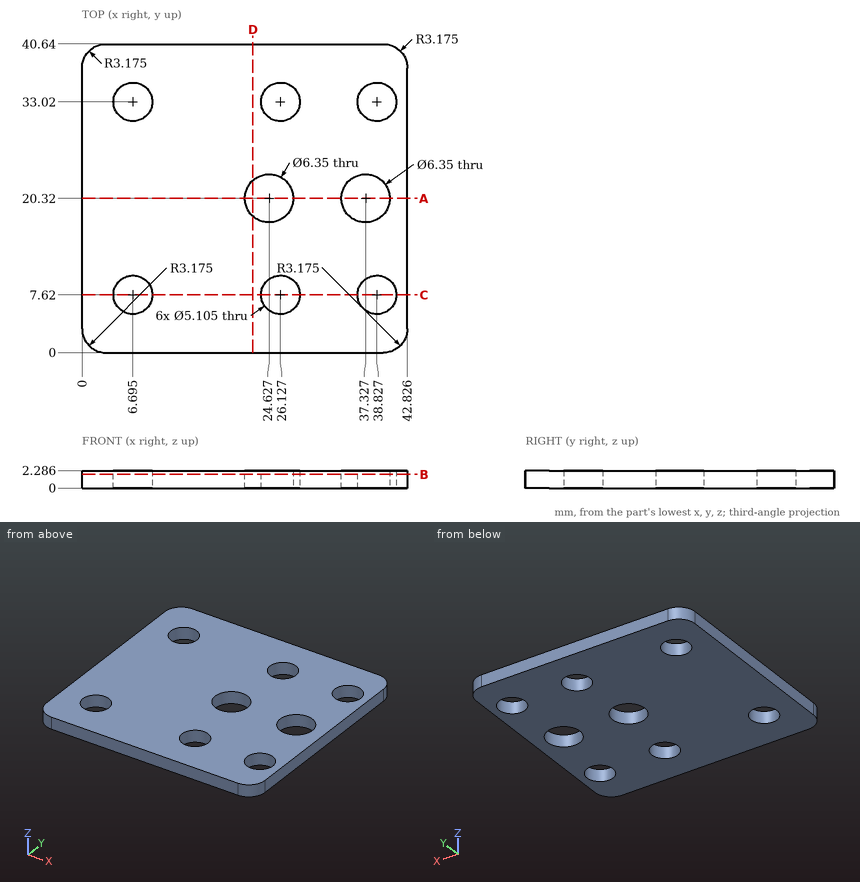
Part print with two shaded views. Sizes in mm from the minimum x, y, z corner. Coordinates: 2 decimals unless noted, no trailing zeros. Write each loop counter-clockwise with the first axis right and the second up, starting at its lowest first coordinate (ties: lowest second). Pieces come first, ordered by that corner, then holes. Notation, with made-up numbers: (-34.5, -34) -> (14.5, -34) arc R16 cw to (14.5, -25) -> close; hole circle Ø11 at (86.5, 44). An arc over 180 degrees is marked (long way). Return JSON: item names as keys, results as strings. Group by question number.
Q1. Cut at B-B, the plane z = 1.8. State how many separate pieces and enclosed holes the cut face has, then the cut area to 3 significant figures.
Q2. Cut at A-A, the plane y = 20.32. Give the cut face in (x, z) (1 decimal).
Q3. Flat gauge pin, fed straight in: pin 1 (3 mm diameter, centred on x = 26.13, y = 33.02, fed in from +Z). Where does the tip first touch, or does it go through?
Q4. Cut at C-C, the plane y = 7.62. Give the cut face in (x, z) (1 decimal).
Q5. Drill centre lines: line 1 (X direction, y = 20.32, z = 1.45) (1 decimal); line 2 (X direction, y = 34.5, z = 1.6) (1 decimal); line 3 (Y direction, x = 27.5, z = 1.9) (1 decimal). Where is each one in solid material? Low to high.
Q6. Cut at D-D, the plane x = 22.5. Give the cut face in (y, z).
Returned:
{
 "1": {"separate pieces": "1", "enclosed holes": "8", "area": "1,550 mm2"},
 "2": {"outline": "(0, 0) -> (21.5, 0) -> (21.5, 2.3) -> (0, 2.3) -> close; (27.8, 0) -> (34.2, 0) -> (34.2, 2.3) -> (27.8, 2.3) -> close; (40.5, 0) -> (42.8, 0) -> (42.8, 2.3) -> (40.5, 2.3) -> close"},
 "3": {"pin 1": "passes through"},
 "4": {"outline": "(0, 0) -> (4.1, 0) -> (4.1, 2.3) -> (0, 2.3) -> close; (9.2, 0) -> (23.6, 0) -> (23.6, 2.3) -> (9.2, 2.3) -> close; (28.7, 0) -> (36.3, 0) -> (36.3, 2.3) -> (28.7, 2.3) -> close; (41.4, 0) -> (42.8, 0) -> (42.8, 2.3) -> (41.4, 2.3) -> close"},
 "5": {"line 1": "x = 0 to 21.5, 27.8 to 34.2, 40.5 to 42.8", "line 2": "x = 0 to 4.6, 8.8 to 24, 28.2 to 36.7, 40.9 to 42.8", "line 3": "y = 0 to 5.5, 9.8 to 19, 21.7 to 30.9, 35.2 to 40.6"},
 "6": {"outline": "(0, 0) -> (17.96, 0) -> (17.96, 2.29) -> (0, 2.29) -> close; (22.68, 0) -> (40.64, 0) -> (40.64, 2.29) -> (22.68, 2.29) -> close"}
}
